Geometry: final body of the model. Coordinates: model frame, mm. Coordinates: 2 decimals unless noted, no trailing zeros. Use CSV: the item, a comma, the result in double quotes. Start each with the question number.
1. First-contact query: P1, Ø5, axis at x = 20.5, z = -4, coming from the +Y side; P2, Ø1, axis at y = 14, z = 5.5, coming from the -X side; P3, Ø1, axis at y = 21, z = 1, coming from the -X side. Flat tips, straight axial feed; report the tip coordinate or a pass-through.
2. Pull-direction query (Z, two-part tool) for faces 1 (the flat face through (12, 20, -9)), 2 (the flat face through (12, 20, 9)); classes: pulls with the +Z half, pulls with the -Z half, needs draft (parallel to the pull), parting line crosses it, or undercut.
3. Material intervals for line 1 (Z direction, x = 1.5, y = 17); line 2 (Y direction, x = 20, z = -3.5); line 3 (X direction, y = 8.5, z = -5.5), sorted ascending.
from build123d import *


with BuildPart() as part:
    # Base → Recubrir3 section 0
    with BuildSketch(Plane.XY):
        Polygon((27.5, 0), (27.5, 40), (12.5, 60), (-2.5, 40), (-2.5, 0), (12.5, -20), align=None)
    # Extrude 2 → Recubrir3 section 1
    with BuildSketch(Plane.XY.offset(9)):
        Polygon((3.5, 38), (3.5, 2), (12.5, -10), (21.5, 2), (21.5, 38), (12.5, 50), align=None)
    loft()

    # Base 2 → Recubrir4 section 0
    with BuildSketch(Plane.XY):
        Polygon((27.5, 0), (27.5, 40), (12.5, 60), (-2.5, 40), (-2.5, 0), (12.5, -20), align=None)
    # Croquis7 → Recubrir4 section 1
    with BuildSketch(Plane(origin=(0, 0, -9), x_dir=(-1, 0, 0), z_dir=(0, 0, -1))):
        Polygon((-21.5, 38), (-12.5, 50), (-3.5, 38), (-3.5, 2), (-12.5, -10), (-21.5, 2), align=None)
    loft()


solid = part.part
Results list:
1,P1,"stops at y = 49.23"
1,P2,"stops at x = 0.83"
1,P3,"stops at x = -2.17"
2,face 1,"pulls with the -Z half"
2,face 2,"pulls with the +Z half"
3,line 1,"z = -6 to 6"
3,line 2,"y = -6.11 to 46.11"
3,line 3,"x = 1.17 to 23.83"
